Here's how the part is built. I have some questions about the finished solid (model axes, mm). Coordinates: 2 decimals unless noted, no trailing zeros. Write each loop counter-clockwise with the first axis right and the second up, starting at its lowest first coordinate (ties: lowest second). Pieces come first, ordered by that corner, then holes. Notation, with made-up numbers: M 2,-4 L 21,-4 A26 ccw 21,19 Z; hole C 28,35.5 d5. An arc over 180 degrees is marked long. Use a Markdown table: item, result.
```python
from build123d import *

# Parameters (mm, degrees)
SKETCH1_W           = 40
SKETCH1_H           = 20
SKETCH1_W_2         = 36
SKETCH1_H_2         = 16
BOSS_EXTRUDE1_DEPTH = 480
CUT_EXTRUDE1_DEPTH  = 483.078831728


with BuildPart() as part:
    # Sketch1 → Boss-Extrude1 (new body)
    with BuildSketch(Plane.XY):
        with Locations((20, -10)):
            Rectangle(SKETCH1_W, SKETCH1_H)
        with Locations((20, -10)):
            Rectangle(SKETCH1_W_2, SKETCH1_H_2, mode=Mode.SUBTRACT)
    extrude(amount=BOSS_EXTRUDE1_DEPTH)

    # Sketch2 → Cut-Extrude1 (cut, through all)
    with BuildSketch(Plane(origin=(40, 0, 0), x_dir=(0, 0, -1), z_dir=(1, 0, 0))):
        Polygon((-480, -20), (-460, 0), (-480, 0), align=None)
        Polygon((-20, 0), (0, 0), (0, -20), align=None)
    extrude(amount=-CUT_EXTRUDE1_DEPTH, mode=Mode.SUBTRACT)


solid = part.part
```
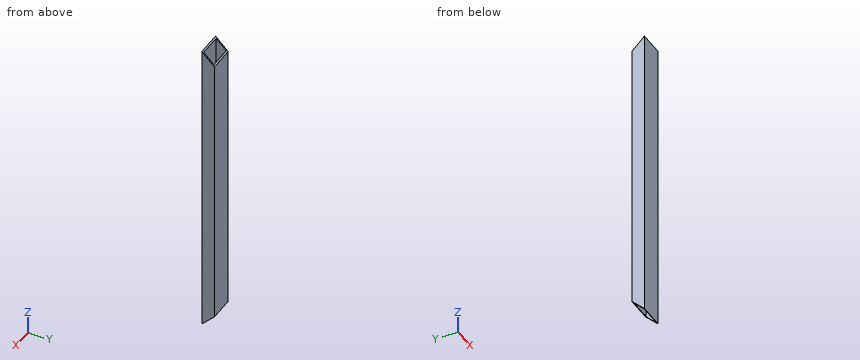
1. I need wall thicknesses on probe 1 along Y at (x, z) = (35.5, 358); probe 2 along X at (y, z) = (-17.25, 227); probe 3 along Z at (x, y) = (16, -18.25). Which ranges of each line are inside material? Lowest first, please.
Answers follow:
| item | result |
|---|---|
| probe 1 | y = -20 to -18, -2 to 0 |
| probe 2 | x = 0 to 2, 38 to 40 |
| probe 3 | z = 1.75 to 478.25 |
2. Suppose I cut it at B-B on y = -7.75. Write out the boundary of the cut face in (x, z), and give its area (3 significant figures).
Answers follow:
| item | result |
|---|---|
| outline | M 0,12.25 L 2,12.25 L 2,467.75 L 0,467.75 Z; M 38,12.25 L 40,12.25 L 40,467.75 L 38,467.75 Z |
| area | 1,820 mm2 |
3. Suppose I cut it at A-A on x = 19.5. Write out the boundary of the cut face in (y, z), and give its area (3 significant figures).
Answers follow:
| item | result |
|---|---|
| outline | M -20,0 L -18,2 L -18,478 L -20,480 Z; M -2,18 L 0,20 L 0,460 L -2,462 Z |
| area | 1,840 mm2 |
4. Suppose I cut it at C-C on z = 306. Write out the boundary of the cut face in (x, y).
Answers follow:
| item | result |
|---|---|
| outline | M 0,-20 L 40,-20 L 40,0 L 0,0 Z; hole M 2,-18 L 38,-18 L 38,-2 L 2,-2 Z |
